from build123d import *

# Parameters (mm, degrees)
EXTRUDE_2_DEPTH          = 50
CUT_EXTRUDE_1_DEPTH      = 154.847326919
CUT_EXTRUDE_1_DEPTH_BACK = 154.847326919
SKETCH_3_R               = 1.65
EXTRUDE_3_DEPTH          = 3
MIRROR_2_COPY_1_DEPTH    = 3
SKETCH_7_R               = 1.65
CUT_EXTRUDE_2_DEPTH      = 10


with BuildPart() as part:
    # 草图1 → 凸台-拉伸2 (new body)
    with BuildSketch(Plane.XY):
        Polygon((-75, 0), (75, 0), (75, -12), (70, -12), (70, -5), (-70, -5), (-70, -12), (-75, -12), align=None)
    extrude(amount=EXTRUDE_2_DEPTH)

    # 草图3 → 切除-拉伸1 (cut, two sides: drawn at the far end of the back side and taken through both)
    with BuildSketch(Plane(origin=(-70, 0, 0), x_dir=(0, 0, -1), z_dir=(1, 0, 0)).offset(-CUT_EXTRUDE_1_DEPTH_BACK)):
        with Locations(Location((-10, -9, 0), (0, 0, 90))):
            Circle(SKETCH_3_R)
        with Locations(Location((-40, -9, 0), (0, 0, 90))):
            Circle(SKETCH_3_R)
    extrude(amount=CUT_EXTRUDE_1_DEPTH + CUT_EXTRUDE_1_DEPTH_BACK, mode=Mode.SUBTRACT)

    # 草图4 → 凸台-拉伸3 (add)
    with BuildSketch(Plane(origin=(0, 0, 0), x_dir=(-1, 0, 0), z_dir=(0, 0, -1))):
        Polygon((64, -5), (70, -12), (70, -5), align=None)
    extrude_3 = extrude(amount=-EXTRUDE_3_DEPTH)

    # 镜向1: 凸台-拉伸3 across plane
    add(extrude_3.mirror(Plane.XY.offset(25)))

    # 镜向2: 凸台-拉伸3 across plane
    add(extrude_3.mirror(Plane(origin=(0, 0, 0), x_dir=(0, 0, 1), z_dir=(1, 0, 0))))

    # 镜向2 copy 1 sketch → 镜向2 copy 1 (add)
    with BuildSketch(Plane.XY.offset(50)):
        Polygon((64, -5), (70, -12), (70, -5), align=None)
    extrude(amount=-MIRROR_2_COPY_1_DEPTH)

    # 草图7 → 切除-拉伸2 (cut)
    with BuildSketch(Plane(origin=(0, 0, 0), x_dir=(1, 0, 0), z_dir=(0, 1, 0))):
        with Locations(Location((50, -35.79, 0), (0, 0, 270))):
            Circle(SKETCH_7_R)
        with Locations(Location((40, -35.79, 0), (0, 0, 270))):
            Circle(SKETCH_7_R)
        with Locations(Location((30, -35.79, 0), (0, 0, 270))):
            Circle(SKETCH_7_R)
        with Locations(Location((20, -35.79, 0), (0, 0, 270))):
            Circle(SKETCH_7_R)
        with Locations(Location((10, -35.79, 0), (0, 0, 270))):
            Circle(SKETCH_7_R)
        with Locations(Location((0, -35.79, 0), (0, 0, 270))):
            Circle(SKETCH_7_R)
        with Locations(Location((-10, -35.79, 0), (0, 0, 270))):
            Circle(SKETCH_7_R)
        with Locations(Location((-20, -35.79, 0), (0, 0, 270))):
            Circle(SKETCH_7_R)
    extrude(amount=-CUT_EXTRUDE_2_DEPTH, mode=Mode.SUBTRACT)


solid = part.part
Check sheet for the modelled part. Datum: model origin and axes. Units: mm. A direction names the side the tool comes from. Give positions to 0.01 mm unless a question says otherwise; leave off trailing zeros. Loops run counter-clockwise (first coordinate to the right, second up) from the corner with the lowest first, then second, coordinate; pieces in that order, holes last. Notation, with made-up numbers: M 86.5,-12 L 103.5,-12 A7 ccw 103.5,-7 Z; hole C 59,20.5 d9. An arc over 180 degrees is marked long. Use a Markdown table: item, result. Add a question column.
Q1. Tool access check on faces 4 (the flat face through (-75, -6, 25)), 5 (the flat face through (68, -7, 47)), 6 (the flat face through (67, -8.5, 1.5)). Record the directions out of +Z, -Z, +X, -X, +Y, -Y that give a thin tool (end or side, any length) a straight path to the whole face; none if there is none.
Q2. Go/stop test with flat-tipped pins: pin 1 (2 mm diameter, centred on x = 30, z = 35.79, fed in from +Y); pin 2 (5.5 mm diameter, centred on x = -10, z = 35.79, fed in from +Y); pin 3 (4.5 mm diameter, centred on x = -20, z = 35.79, fed in from -Y). Record where each tip stops, or that it passes through.
Q3. Sectioned sample at C-C, the plane y = -9.25. Give the number of separate pieces and of enclosed holes in the cut face, then the cut area to 3 significant figures.
Q4. Scan lines: line 1 along Z through (x, y) = (72.35, -9); line 2 along X through (y, z) = (-6.5, 11.5); line 3 along Y through (x, z) = (-72.65, 10). Record each from-to range of solid material in increasing order. Write a range as [from, to].
Q5. Mould release check, pull along Y, two halves, no side actions. Record for faces 1 (the cylindrical face through (72.465, -9.215, 41.636)), 2 (the flat face through (73, -12, 25)), 3 (the flat face through (-68, -7, 47)): pulls with the +Y half, pulls with the -Y half, needs draft (parallel to the pull), parting line crosses it, or undercut.
Q6. Sectioned sample at B-B, the plane x = 10. Record the cut outline in (y, z), then the cut area to 4 significant figures.
Q7. Sectioned sample at A-A, the plane z = 10. Record the cut outline in (x, y), then the cut area to 3 significant figures.
Verdict:
| question | item | result |
|---|---|---|
| 1 | face 4 | +Z, -Z, -X, +Y, -Y |
| 1 | face 5 | -Y |
| 1 | face 6 | +Z, -Z, -Y |
| 2 | pin 1 | through |
| 2 | pin 2 | y = 0 |
| 2 | pin 3 | y = -5 |
| 3 | separate pieces | 6 |
| 3 | enclosed holes | 0 |
| 3 | area | 463 mm^2 |
| 4 | line 1 | [0, 8.35], [11.65, 38.35], [41.65, 50] |
| 4 | line 2 | [-75, -70], [70, 75] |
| 4 | line 3 | [-12, -10.65], [-7.35, 0] |
| 5 | face 1 | undercut |
| 5 | face 2 | pulls with the -Y half |
| 5 | face 3 | needs draft |
| 6 | outline | M -5,0 L 0,0 L 0,34.14 L -5,34.14 Z; M -5,37.44 L 0,37.44 L 0,50 L -5,50 Z |
| 6 | area | 233.5 mm^2 |
| 7 | outline | M -75,-12 L -70,-12 L -70,-10.65 L -75,-10.65 Z; M -75,-7.35 L -70,-7.35 L -70,-5 L 70,-5 L 70,-7.35 L 75,-7.35 L 75,0 L -75,0 Z; M 70,-12 L 75,-12 L 75,-10.65 L 70,-10.65 Z |
| 7 | area | 787 mm^2 |
